Solid Edge part; units mm, degrees
sketch "Sketch1" plane through (0, 0, 58.4958) normal (0, 0, 1) x (1, 0, 0)
  line L0 (-58, 76.5) -> (-23, 76.5)
  line L1 (-23, 76.5) -> (-23, 111.5)
  line L2 (-23, 111.5) -> (-58, 111.5)
  line L3 (-58, 111.5) -> (-58, 76.5)
extrude "Protrusion1" add sketch "Sketch1" along normal blind 20
fillet "Round_1" radius 3 4 edges at (-23, 111.5, 68.4958) (-58, 111.5, 68.4958) (-58, 76.5, 68.4958) (-23, 76.5, 68.4958)
chamfer "Chamfer_3" distance 2 angle 45 15 edges at (-58, 94, 78.4958) (-57.1213, 77.3787, 78.4958) (-40.5, 76.5, 78.4958) (-23.8787, 77.3787, 78.4958) (-23, 94, 78.4958) (-23.8787, 110.6213, 78.4958) (-40.5, 111.5, 78.4958) (-57.1213, 110.6213, 78.4958) (-58, 94, 58.4958) (-57.1213, 77.3787, 58.4958) (-40.5, 76.5, 58.4958) (-23.8787, 77.3787, 58.4958) (-23, 94, 58.4958) (-40.5, 111.5, 58.4958) (-57.1213, 110.6213, 58.4958)
sketch "Sketch2" plane through (-40.5, 76.5, 65.9958) normal (0, -1, 0) x (1, 0, 0)
  circle A0 centre (0, 2.5) radius 2.65
extrude "ExtrudedCutout_1" cut sketch "Sketch2" against normal blind 2.3
sketch "Sketch3" plane through (-40.5, 111.5, 65.9958) normal (0, 1, 0) x (-1, 0, 0)
  circle A0 centre (0, 2.5) radius 2.65
extrude "ExtrudedCutout_4" cut sketch "Sketch3" against normal blind 2.3
sketch "Sketch4" plane through (-58, 94, 65.9958) normal (-1, 0, 0) x (0, -1, 0)
  circle A0 centre (0, 2.5) radius 2.65
extrude "ExtrudedCutout_5" cut sketch "Sketch4" against normal blind 2.3
sketch "Sketch5" plane through (-23, 94, 65.9958) normal (1, 0, 0) x (0, 1, 0)
  circle A0 centre (0, 2.5) radius 2.65
extrude "ExtrudedCutout_6" cut sketch "Sketch5" against normal blind 2.3
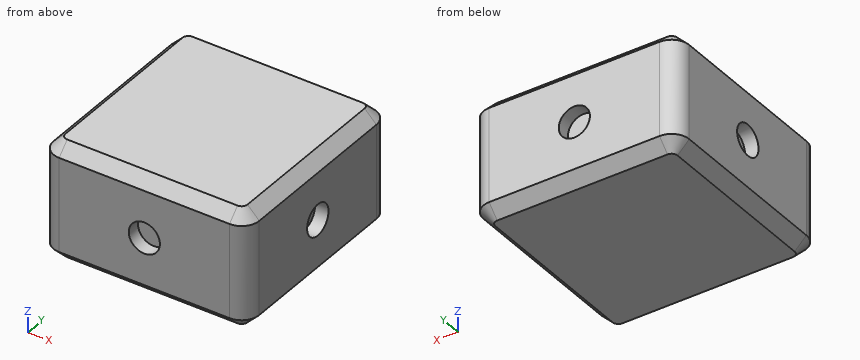
For this review, take the finished solid that the model builds, in its own axes (mm). Round coordinates to 2 decimals unless told otherwise and drop trailing zeros. Loops run counter-clockwise (first coordinate to the right, second up) from the corner with the lowest first, then second, coordinate; pieces in that order, holes last.
Q1. Insertion check: pin 1 Ø4 at (x, z) = (-40.5, 68) entering from -Y; pin 2 Ø4 at (y, z) = (94, 68.5) entering from +X; pin 3 Ø5 at (x, z) = (-40.5, 68.5) entering from +Y. Each pin has a flat end and moves straight along its axis. Give the tip position at first contact, or say it passes through.
Result sheet:
pin 1: stops at y = 78.8
pin 2: stops at x = -25.3
pin 3: stops at y = 109.2
Q2. Add section B-B on y = 94. Write out the cut boundary in (x, z).
Result sheet:
outline: (-58, 60.5) - (-56, 58.5) - (-25, 58.5) - (-23, 60.5) - (-23, 65.85) - (-25.3, 65.85) - (-25.3, 71.15) - (-23, 71.15) - (-23, 76.5) - (-25, 78.5) - (-56, 78.5) - (-58, 76.5) - (-58, 71.15) - (-55.7, 71.15) - (-55.7, 65.85) - (-58, 65.85) - close
Q3. To check wall thickness, follow line 1 along Z through (x, y) = (-40, 77); line 2 along Z through (x, y) = (-40.5, 110.4); line 3 along X through (y, z) = (79, 74.5). State the ranges of each line that lie inside material, in increasing order.
Result sheet:
line 1: z = 60 to 65.89, 71.1 to 77
line 2: z = 59.4 to 65.85, 71.15 to 77.6
line 3: x = -57.96 to -23.04
Q4. Add section A-A on x = -40.5. Write out the cut boundary in (y, z).
Result sheet:
outline: (76.5, 60.5) - (78.5, 58.5) - (109.5, 58.5) - (111.5, 60.5) - (111.5, 65.85) - (109.2, 65.85) - (109.2, 71.15) - (111.5, 71.15) - (111.5, 76.5) - (109.5, 78.5) - (78.5, 78.5) - (76.5, 76.5) - (76.5, 71.15) - (78.8, 71.15) - (78.8, 65.85) - (76.5, 65.85) - close
